Source: CAD feature listing. Evaluate the final solid. Frame: model axes, mm. Face numbers are marked on the shaded views. A direction names the side the tool comes from. Give positions to 0.01 mm unless a question says otherwise; leave off trailing zeros. Loops run counter-clockwise (first coordinate to the right, second up) from the corner with the lowest first, then second, coordinate; pieces in that order, holes last. Notation, with made-up numbers: (78, 82.25) -> (131, 82.25) arc R19 cw to (131, 92.25) -> close; hole circle Ø2 at (-33, 30.25). An arc over 180 degrees is marked (long way). Put each result on its own line as item: value.
```python
from build123d import *

# Parameters (mm, degrees)
CROQUIS2_W            = 5
CROQUIS2_H            = 39.415776956
CORTAR_EXTRUIR1_DEPTH = 22.5
MATRIZC2_COUNT        = 3
MATRIZC2_ANGLE        = 180
CROQUIS3_R            = 13.25
CORTAR_EXTRUIR2_DEPTH = 32
REDONDEO2_R           = 10
CHAFL_N1_SIZE         = 0.5
CHAFL_N2_SIZE         = 2
CROQUIS4_R            = 9
CORTAR_EXTRUIR3_DEPTH = 139.767791652
CROQUIS4_3_R          = 13.5
CROQUIS4_3_R_2        = 9
CORTAR_EXTRUIR4_DEPTH = 97


# Some blends are built 0.0001 mm under size
with BuildPart() as part:
    # Croquis1 → Revolución1 (revolve)
    with BuildSketch(Plane(origin=(0, 0, 0), x_dir=(0, 0, -1), z_dir=(1, 0, 0))):
        Polygon((0, 0), (-15.25, 0), (-15.25, 11), (-16, 11), (-16, 16), (-14.5, 16), (-14.5, 57), (-16.25, 57), (-16.25, 62), (-14.75, 62), (-14.75, 63), (-16.25, 63), (-16.25, 69), (-16, 69), (-16, 80), (-16.75, 80), (-16.75, 84), (-17.5, 84), (-17.5, 91), (-19.5, 91), (-19.5, 94), (-17.5, 94), (-17.5, 104), (-15.75, 104), (-15.75, 136), (0, 136), align=None)
    revolve(axis=Axis((0, 136, 0), (0, -1, 0)))

    # Croquis2 → Cortar-Extruir1 (cut, symmetric)
    with BuildSketch(Plane(origin=(0, 0, 0), x_dir=(0, 0, -1), z_dir=(1, 0, 0))):
        with Locations((0, 123.707888478)):
            Rectangle(CROQUIS2_W, CROQUIS2_H)
    cortar_extruir1 = extrude(amount=CORTAR_EXTRUIR1_DEPTH, both=True, mode=Mode.SUBTRACT)

    # MatrizC2: Cortar-Extruir1 ×3 about axis
    matrizc2_axis = Axis((0, 136, 0), (0, 1, 0))
    for i in range(1, MATRIZC2_COUNT):
        add(cortar_extruir1.rotate(matrizc2_axis, i * MATRIZC2_ANGLE / (MATRIZC2_COUNT - 1)), mode=Mode.SUBTRACT)

    # Croquis3 → Cortar-Extruir2 (cut)
    with BuildSketch(Plane(origin=(0, 136, 0), x_dir=(1, 0, 0), z_dir=(0, 1, 0))):
        Circle(CROQUIS3_R)
    extrude(amount=-CORTAR_EXTRUIR2_DEPTH, mode=Mode.SUBTRACT)

    # Redondeo2
    # the kernel refuses this fillet: 10 mm, written as the material it adds along each edge
    with BuildSketch(Plane(origin=(0, 91, 0), x_dir=(0, 0, 1), z_dir=(1, 0, 0))) as redondeo2_piece_1:
        with BuildLine():
            CenterArc((27.5, 6), REDONDEO2_R, 180, 36.869897646)
            Line((19.5, 0), (17.5, 0))
            Line((17.5, 0), (17.5, 6))
        make_face()
    revolve(axis=Axis((0, 91, 0), (0, -1, 0)))

    # Chaflán1
    chafl_n1_edges = [part.edges().sort_by_distance(p)[0] for p in [
        (0, 63, -14.75),
        (0, 62, -14.75),
        (0, 11, -15.25),
    ]]
    chamfer(chafl_n1_edges, length=CHAFL_N1_SIZE - 0.0001)  # a hair under: the kernel refuses the full size

    # Chaflán2
    # the kernel refuses this chamfer: 2 mm, written as the material it adds along each edge
    with BuildSketch(Plane(origin=(0, 16, 0), x_dir=(0, 0, 1), z_dir=(1, 0, 0))) as chafl_n2_piece_1_section:
        Polygon((14.5, -CHAFL_N2_SIZE), (14.5 + CHAFL_N2_SIZE, 0), (14.5, 0), align=None)
    chafl_n2_piece_1 = revolve(axis=Axis((0, 16, 0), (0, -1, 0)), mode=Mode.PRIVATE)
    chafl_n2_piece_1 = chafl_n2_piece_1 & Plane(origin=(0, 16, 0), x_dir=(0, 0, 1), z_dir=(0, 1, 0)) * Cylinder(16, 66, mode=Mode.PRIVATE)
    add(chafl_n2_piece_1)
    with BuildSketch(Plane(origin=(0, 57, 0), x_dir=(0, 0, 1), z_dir=(1, 0, 0))) as chafl_n2_piece_2_section:
        Polygon((14.5 + CHAFL_N2_SIZE, 0), (14.5, CHAFL_N2_SIZE), (14.5, 0), align=None)
    chafl_n2_piece_2 = revolve(axis=Axis((0, 57, 0), (0, -1, 0)), mode=Mode.PRIVATE)
    chafl_n2_piece_2 = chafl_n2_piece_2 & Plane(origin=(0, 57, 0), x_dir=(0, 0, 1), z_dir=(0, 1, 0)) * Cylinder(16.25, 66, mode=Mode.PRIVATE)
    add(chafl_n2_piece_2)

    # Croquis4 → Cortar-Extruir3 (cut, through all)
    with BuildSketch(Plane.XZ):
        with Locations(Location((0, 0, 0), (0, 0, 270))):
            Circle(CROQUIS4_R)
    extrude(amount=-CORTAR_EXTRUIR3_DEPTH, mode=Mode.SUBTRACT)

    # Croquis4<3> → Cortar-Extruir4 (cut)
    with BuildSketch(Plane.XZ):
        with Locations(Location((0, 0, 0), (0, 0, 270))):
            Circle(CROQUIS4_3_R)
        with Locations(Location((0, 0, 0), (0, 0, 90))):
            Circle(CROQUIS4_3_R_2, mode=Mode.SUBTRACT)
    extrude(amount=-CORTAR_EXTRUIR4_DEPTH, mode=Mode.SUBTRACT)

    # Croquis6 → Cortar-Revolución1 (revolve, cut)
    with BuildSketch(Plane(origin=(0, 0, 0), x_dir=(0, 0, -1), z_dir=(1, 0, 0)), mode=Mode.PRIVATE) as cortar_revoluci_n1_sk:
        Polygon((16, 79.5), (13.766586279, 79), (3.766586279, 79), (3.766586279, 76.5), (-16, 76.5), (-16, 74.5), (16, 74.5), align=None)
    revolve(cortar_revoluci_n1_sk.sketch.rotate(Axis((0, 74.5, 16), (0, 0, -1)), 90), axis=Axis((0, 74.5, 16), (0, 0, -1)), mode=Mode.SUBTRACT)


solid = part.part
```
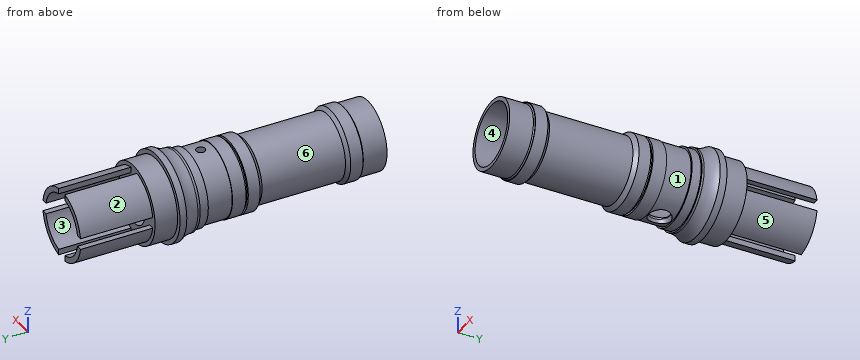
(1) Section B-B on y = 74.5. Return loops of the section in (x, z).
Calculated:
outline: (-4.83, -15.25) -> (-4.5, -13.77) -> (-4.5, -12.73) arc R13.5 cw to (-2, 13.35) -> (-2, 15.87) arc R16 ccw to start; (2, 13.35) arc R13.5 cw to (4.5, -12.73) -> (4.5, -13.77) -> (4.83, -15.25) arc R16 ccw to (2, 15.87) -> close
(2) Section A-A on x = 0. Give the number of separate pieces and of enclosed holes in the cut face, then the cut area to 3 significant figures.
Calculated:
separate pieces: 4
enclosed holes: 0
area: 507 mm²
(3) Section D-D on y = 34. Return loops of the section in (x, z).
Calculated:
outline: circle Ø29 at (0, 0); hole circle Ø27 at (0, 0)
(4) First-contact query: P1, Ø0.8, axis at y = 116, z = -14.5, coming from the -X side; P2, Ø1, axis at y = 65, z = 15, coming from the +X side; P3, Ø0.8, axis at y = 127, z = 13.5, coming from the +X side; P4, Ø11, axis at x = 0, z = 0, coming from the -Y side. Flat tips, straight axial feed; report the tip coordinate or a pass-through.
Calculated:
P1: stops at x = -7.02
P2: stops at x = 7.34
P3: stops at x = 8.74
P4: passes through
(5) Reachability of the marked faces 1, 2, 3 and 4 from +Z, -Z, +X, -X, +Y, -Y: full face, straight path, thin tool, end or side. Return the list, or none.
Calculated:
face 1: none
face 2: +Z, -X, +Y
face 3: +Y
face 4: -Y
(6) Line query: probe 1 along X at (y, z) = (100, 0); probe 2 along X at (y, z) = (55, 0). Output: solid intervals per line, ascending. Write a range as from..to.
Calculated:
probe 1: x = -17.5..-9, 9..17.5
probe 2: x = -14.5..-13.5, 13.5..14.5
(7) Section C-C on y = 9. Return loops of the section in (x, z).
Calculated:
outline: circle Ø30.5 at (0, 0); hole circle Ø27 at (0, 0)
(8) Draft query along Y for the marked faces 5 and 6. Return one class per face: released by +Y, released by -Y, zero draft, split by the parting line, or undercut.
Calculated:
face 5: zero draft
face 6: undercut
